Geometry: final body of the model. Coordinates: model frame, mm. A direction names the side the tool comes from. Round coordinates to 2 decimals unless told otherwise and drop trailing zeros. Loops run counter-clockwise (first coordinate to the right, second up) from the corner with the lowest first, then second, coordinate; pieces in that order, holes last. Notation, with made-up numbers: (62, 21.5) - (119, 21.5) arc R8 ccw to (119, 27.5) - close; hole circle Ø5 at (59.25, 87). An arc over 180 degrees is marked (long way). Answer as a JSON object with one key per item and string values. Group by question number.
Item 1: Section D-D (y = -12.5). Return the cut outline in (x, z).
Item 2: Draft query along X for faces 4 (the face through (4, 5, 24.7)), 5 (the face through (38, -30, 56)), 6 (the face through (45, -17, 32)). Return one class per face: released by +X, released by -X, zero draft, split by the parting line, or undercut.
Item 3: Reachability of faces 1 (the face through (40.545, -30.479, 3.774)), 2 (the face through (22, 0, 47)), 3 (the face through (41, 5, 24.7)) from +Z, -Z, +X, -X, +Y, -Y: full face, straight path, thin tool, end or side. Return the list, or none.
Item 4: First-contact query: pin 1 (3 mm diameter, centred on x = 37, z = 40.5, fed in from +Y); pin 2 (2 mm diameter, centred on x = 41, y = 6.5, fed in from +Z); pin 3 (10 mm diameter, centred on x = 24, y = 3, fed in from -Z). Flat tips, straight axial feed; report the tip coordinate or a pass-through.
Item 5: Line query: line 1 (Z direction, x = 30, y = -25.5); line 2 (Z direction, x = 24, y = -12); line 3 (Z direction, x = 43.5, y = 8). Output: solid intervals per line, ascending.
Item 6: Section A-A (y = 6). Return the cut outline in (x, z).
Item 7: Section C-C (x = 17.5). Count the separate pieces of the cut face and the enclosed holes in it, plus the area to 3 significant figures.
Item 8: Section B-B (z = 52.5). Return the cut outline in (x, y), plus the area to 3 significant figures.
```python
from build123d import *

# Parameters (mm, degrees)
SKETCH_W        = 45
SKETCH_H        = 65
PAD_DEPTH       = 35
SKETCH001_R     = 7.5
POCKET_DEPTH    = 45.001
SKETCH002_R     = 2
POCKET001_DEPTH = 6
SKETCH003_W     = 8
SKETCH003_H     = 4
POCKET002_DEPTH = 45.001
POCKET003_DEPTH = 3
SKETCH005_R     = 3
SKETCH005_W     = 45
SKETCH005_H     = 4.8
PAD001_DEPTH    = 10
CHAMFER_SIZE    = 1
CHAMFER001_SIZE = 3
CHAMFER002_SIZE = 2


with BuildPart() as part:
    # Sketch → Pad (new body)
    with BuildSketch(Plane.XZ):
        with Locations((22.5, 32.5)):
            Rectangle(SKETCH_W, SKETCH_H)
    extrude(amount=PAD_DEPTH)

    # Sketch001 (on Face2 of Pad) → Pocket (cut, through all)
    with BuildSketch(Plane(origin=(45, 0, 0), x_dir=(0, 0, 1), z_dir=(1, 0, 0))):
        with Locations((52.5, 12.5)):
            Circle(SKETCH001_R)
        with Locations((12.5, 12.5)):
            Circle(SKETCH001_R)
    extrude(amount=-POCKET_DEPTH, mode=Mode.SUBTRACT)

    # Sketch002 (on Face6 of Pad) → Pocket001 (cut)
    with BuildSketch(Plane.XZ.offset(35)):
        with Locations((7.5, 59.5)):
            Circle(SKETCH002_R)
        with Locations((37.5, 59.5)):
            Circle(SKETCH002_R)
        with Locations((7.5, 5.5)):
            Circle(SKETCH002_R)
        with Locations((37.5, 5.5)):
            Circle(SKETCH002_R)
    extrude(amount=-POCKET001_DEPTH, mode=Mode.SUBTRACT)

    # Sketch003 (on Face3 of Pocket001) → Pocket002 (cut, through all)
    with BuildSketch(Plane(origin=(45, 0, 0), x_dir=(0, 0, 1), z_dir=(1, 0, 0))):
        with Locations((5.5, 27)):
            Rectangle(SKETCH003_W, SKETCH003_H)
        with Locations((59.5, 27)):
            Rectangle(SKETCH003_W, SKETCH003_H)
    extrude(amount=-POCKET002_DEPTH, mode=Mode.SUBTRACT)

    # Sketch004 (on Face14 of Pocket002) → Pocket003 (cut)
    with BuildSketch(Plane(origin=(0, -29, 0), x_dir=(1, 0, 0), z_dir=(0, 1, 0))):
        Polygon((11.541452, -5.5), (9.520726, -2), (5.479274, -2), (3.458548, -5.5), (5.479274, -9), (9.520726, -9), align=None)
        Polygon((39.520726, -9), (41.541452, -5.5), (39.520726, -2), (35.479274, -2), (33.458548, -5.5), (35.479274, -9), align=None)
        Polygon((9.520726, -63), (11.541452, -59.5), (9.520726, -56), (5.479274, -56), (3.458548, -59.5), (5.479274, -63), align=None)
        Polygon((39.520726, -63), (41.541452, -59.5), (39.520726, -56), (35.479274, -56), (33.458548, -59.5), (35.479274, -63), align=None)
    extrude(amount=-POCKET003_DEPTH, mode=Mode.SUBTRACT)

    # Sketch005 (on Face4 of Pocket003) → Pad001 (join)
    with BuildSketch(Plane(origin=(0, 0, 0), x_dir=(1, 0, 0), z_dir=(0, 1, 0))):
        with Locations((27.5, -22.7)):
            Circle(SKETCH005_R)
        with Locations((17.5, -22.7)):
            Circle(SKETCH005_R)
        Polygon((45, -24.7), (45, -12.7), (0, -12.7), (0, -24.7), (7.5, -24.7), (14.5, -17.7), (30.5, -17.7), (37.5, -24.7), align=None)
        with Locations((22.5, -30.1)):
            Rectangle(SKETCH005_W, SKETCH005_H)
    extrude(amount=PAD001_DEPTH)

    # Chamfer
    chamfer_edges = [part.edges().sort_by_distance(p)[0] for p in [
        (22.5, -35, 65),
        (22.5, -35, 0),
    ]]
    chamfer(chamfer_edges, length=CHAMFER_SIZE)

    # Chamfer001
    chamfer001_edges = [part.edges().sort_by_distance(p)[0] for p in [
        (22.5, 0, 65),
        (22.5, 0, 0),
    ]]
    chamfer(chamfer001_edges, length=CHAMFER001_SIZE)

    # Chamfer002
    chamfer002_edges = [part.edges().sort_by_distance(p)[0] for p in [
        (22.5, 10, 32.5),
        (22.5, 10, 12.7),
    ]]
    chamfer(chamfer002_edges, length=CHAMFER002_SIZE)


solid = part.part
```
Values:
{
 "1": {"outline": "(0, 0) - (45, 0) - (45, 5) - (0, 5) - close; (0, 20) - (45, 20) - (45, 45) - (0, 45) - close; (0, 60) - (45, 60) - (45, 65) - (0, 65) - close"},
 "2": {"face 4": "zero draft", "face 5": "undercut", "face 6": "released by +X"},
 "3": {"face 1": "none", "face 2": "+Z, +X, -X, +Y", "face 3": "+X, +Y"},
 "4": {"pin 1": "stops at y = 0", "pin 2": "stops at z = 32.5", "pin 3": "stops at z = 1"},
 "5": {"line 1": "z = 0 to 1.5, 9.5 to 55.5, 63.5 to 65", "line 2": "z = 0 to 5.02, 19.98 to 45.02, 59.98 to 65", "line 3": "z = 12.7 to 24.7, 27.7 to 32.5"},
 "6": {"outline": "(0, 12.7) - (45, 12.7) - (45, 24.7) - (37.5, 24.7) - (30.5, 17.7) - (14.5, 17.7) - (7.5, 24.7) - (0, 24.7) - close; (0, 27.7) - (45, 27.7) - (45, 32.5) - (0, 32.5) - close; circle Ø6 at (17.5, 22.7); circle Ø6 at (27.5, 22.7)"},
 "7": {"separate pieces": "1", "enclosed holes": "4", "area": "2,000 mm^2"},
 "8": {"outline": "(0, -35) - (45, -35) - (45, -20) - (0, -20) - close; (0, -5) - (45, -5) - (45, 0) - (0, 0) - close", "area": "900 mm^2"}
}
